For this review, take the finished solid that the model builds, in its own axes (mm). Face numbers are marked on the shaded views. A direction names the side the tool comes from. Coordinates: 2 decimals unless noted, no trailing zeros. Order: outer loops, then holes, each group sorted by start corner. A loop starts at its lowest first (then second) coordinate and runs counter-clockwise, first axis right, second up. Notation, with made-up numbers: M 37,10.5 L 59,10.5 A27 cw 59,46.5 Z; hole C 61,33 d11. An arc over 180 degrees is marked long. Use CSV: the item, a comma, the result in double quotes.
```python
from build123d import *

# Parameters (mm, degrees)
SKETCH2_R                            = 3.35
F_40_SERIES_TS40_40LM_650033_2_DEPTH = 115
M8X1_25_TAPPED_HOLE3_D               = 6.8
M8X1_25_TAPPED_HOLE3_DEPTH           = 25
M8X1_25_TAPPED_HOLE3_TIP             = 2.042926105


with BuildPart() as part:
    # Sketch2 → 40 series TS40-40LM-650033(2) (new body)
    with BuildSketch(Plane(origin=(0, 0, 0), x_dir=(-1, 0, 0), z_dir=(0, 1, 0))):
        with BuildLine():
            Line((-7.7064, 0), (-7.7064, 5.551138531))
            Line((-7.7064, 5.551138531), (-13.331261469, 11.176))
            Line((-13.331261469, 11.176), (-16.6472, 11.176))
            Line((-16.6472, 11.176), (-16.6472, 7.6835))
            Line((-16.6472, 7.6835), (-15.2502, 7.6835))
            Line((-15.2502, 7.6835), (-15.2502, 4.0005))
            Line((-15.2502, 4.0005), (-20, 4.0005))
            Line((-20, 4.0005), (-20, 16.825))
            ThreePointArc((-20, 16.825), (-19.07006403, 19.07006403), (-16.825, 20))
            Line((-16.825, 20), (-4.0005, 20))
            Line((-4.0005, 20), (-4.0005, 15.2502))
            Line((-4.0005, 15.2502), (-7.6835, 15.2502))
            Line((-7.6835, 15.2502), (-7.6835, 16.6472))
            Line((-7.6835, 16.6472), (-11.176, 16.6472))
            Line((-11.176, 16.6472), (-11.176, 13.331261469))
            Line((-11.176, 13.331261469), (-5.551138531, 7.7064))
            Line((-5.551138531, 7.7064), (0, 7.7064))
            Line((0, 7.7064), (5.551138531, 7.7064))
            Line((5.551138531, 7.7064), (11.176, 13.331261469))
            Line((11.176, 13.331261469), (11.176, 16.6472))
            Line((11.176, 16.6472), (7.6835, 16.6472))
            Line((7.6835, 16.6472), (7.6835, 15.2502))
            Line((7.6835, 15.2502), (4.0005, 15.2502))
            Line((4.0005, 15.2502), (4.0005, 20))
            Line((4.0005, 20), (16.825, 20))
            ThreePointArc((16.825, 20), (19.07006403, 19.07006403), (20, 16.825))
            Line((20, 16.825), (20, 4.0005))
            Line((20, 4.0005), (15.2502, 4.0005))
            Line((15.2502, 4.0005), (15.2502, 7.6835))
            Line((15.2502, 7.6835), (16.6472, 7.6835))
            Line((16.6472, 7.6835), (16.6472, 11.176))
            Line((16.6472, 11.176), (13.331261469, 11.176))
            Line((13.331261469, 11.176), (7.7064, 5.551138531))
            Line((7.7064, 5.551138531), (7.7064, 0))
            Line((7.7064, 0), (7.7064, -5.551138531))
            Line((7.7064, -5.551138531), (13.331261469, -11.176))
            Line((13.331261469, -11.176), (16.6472, -11.176))
            Line((16.6472, -11.176), (16.6472, -7.6835))
            Line((16.6472, -7.6835), (15.2502, -7.6835))
            Line((15.2502, -7.6835), (15.2502, -4.0005))
            Line((15.2502, -4.0005), (20, -4.0005))
            Line((20, -4.0005), (20, -16.825))
            ThreePointArc((20, -16.825), (19.07006403, -19.07006403), (16.825, -20))
            Line((16.825, -20), (4.0005, -20))
            Line((4.0005, -20), (4.0005, -15.2502))
            Line((4.0005, -15.2502), (7.6835, -15.2502))
            Line((7.6835, -15.2502), (7.6835, -16.6472))
            Line((7.6835, -16.6472), (11.176, -16.6472))
            Line((11.176, -16.6472), (11.176, -13.331261469))
            Line((11.176, -13.331261469), (5.551138531, -7.7064))
            Line((5.551138531, -7.7064), (0, -7.7064))
            Line((0, -7.7064), (-5.551138531, -7.7064))
            Line((-5.551138531, -7.7064), (-11.176, -13.331261469))
            Line((-11.176, -13.331261469), (-11.176, -16.6472))
            Line((-11.176, -16.6472), (-7.6835, -16.6472))
            Line((-7.6835, -16.6472), (-7.6835, -15.2502))
            Line((-7.6835, -15.2502), (-4.0005, -15.2502))
            Line((-4.0005, -15.2502), (-4.0005, -20))
            Line((-4.0005, -20), (-16.825, -20))
            ThreePointArc((-16.825, -20), (-19.07006403, -19.07006403), (-20, -16.825))
            Line((-20, -16.825), (-20, -4.0005))
            Line((-20, -4.0005), (-15.2502, -4.0005))
            Line((-15.2502, -4.0005), (-15.2502, -7.6835))
            Line((-15.2502, -7.6835), (-16.6472, -7.6835))
            Line((-16.6472, -7.6835), (-16.6472, -11.176))
            Line((-16.6472, -11.176), (-13.331261469, -11.176))
            Line((-13.331261469, -11.176), (-7.7064, -5.551138531))
            Line((-7.7064, -5.551138531), (-7.7064, 0))
        make_face()
        Circle(SKETCH2_R, mode=Mode.SUBTRACT)
        with BuildLine():
            Line((18.222, 12.8372), (18.222, 15.428))
            ThreePointArc((18.222, 15.428), (17.403656347, 17.403656347), (15.428, 18.222))
            Line((15.428, 18.222), (12.8372, 18.222))
            Line((12.8372, 18.222), (12.8372, 12.8372))
            Line((12.8372, 12.8372), (18.222, 12.8372))
        make_face(mode=Mode.SUBTRACT)
        with BuildLine():
            Line((12.8372, -12.8372), (18.222, -12.8372))
            Line((18.222, -12.8372), (18.222, -15.428))
            ThreePointArc((18.222, -15.428), (17.403656347, -17.403656347), (15.428, -18.222))
            Line((15.428, -18.222), (12.8372, -18.222))
            Line((12.8372, -18.222), (12.8372, -12.8372))
        make_face(mode=Mode.SUBTRACT)
        with BuildLine():
            Line((-18.222, -12.8372), (-18.222, -15.428))
            ThreePointArc((-18.222, -15.428), (-17.403656347, -17.403656347), (-15.428, -18.222))
            Line((-15.428, -18.222), (-12.8372, -18.222))
            Line((-12.8372, -18.222), (-12.8372, -12.8372))
            Line((-12.8372, -12.8372), (-18.222, -12.8372))
        make_face(mode=Mode.SUBTRACT)
        with BuildLine():
            Line((-12.8372, 12.8372), (-18.222, 12.8372))
            Line((-18.222, 12.8372), (-18.222, 15.428))
            ThreePointArc((-18.222, 15.428), (-17.403656347, 17.403656347), (-15.428, 18.222))
            Line((-15.428, 18.222), (-12.8372, 18.222))
            Line((-12.8372, 18.222), (-12.8372, 12.8372))
        make_face(mode=Mode.SUBTRACT)
    extrude(amount=F_40_SERIES_TS40_40LM_650033_2_DEPTH)

    # M8x1.25 Tapped Hole3
    with Locations(Plane(origin=(0, 0, 0), x_dir=(-1, 0, 0), z_dir=(0, -1, 0))):
        with Locations((0, 0)):
            Hole(M8X1_25_TAPPED_HOLE3_D / 2, depth=M8X1_25_TAPPED_HOLE3_DEPTH)
            with Locations((0, 0, -(M8X1_25_TAPPED_HOLE3_DEPTH + M8X1_25_TAPPED_HOLE3_TIP / 2))):  # 118° drill point
                Cone(0, M8X1_25_TAPPED_HOLE3_D / 2, M8X1_25_TAPPED_HOLE3_TIP, mode=Mode.SUBTRACT)


solid = part.part
```
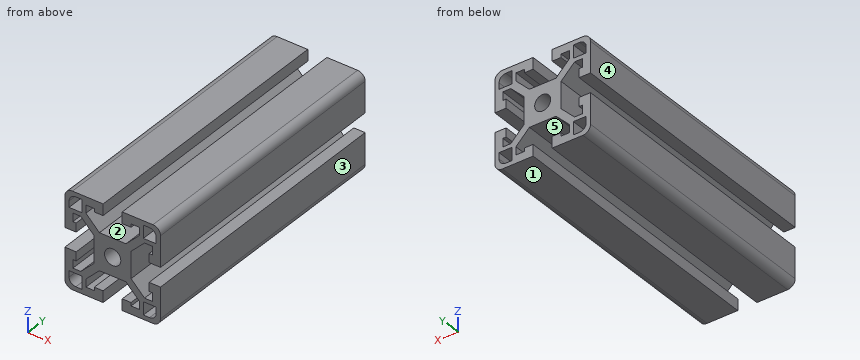
Item 1: Add section D-D on z = 10. State the section outline as (x, y) points, and give its area (3 significant figures).
Solutions:
outline,"M -20,0 L -16.65,0 L -16.65,115 L -20,115 Z; M -12.16,0 L -7.84,0 L -7.84,115 L -12.16,115 Z; M 7.84,0 L 12.16,0 L 12.16,115 L 7.84,115 Z; M 16.65,0 L 20,0 L 20,115 L 16.65,115 Z"
area,"1,760 mm^2"
Item 2: Add section A-A on z = 0. State the section outline as (x, y) points, and give its area (3 significant figures).
Solutions:
outline,"M -7.71,0 L -3.4,0 L -3.4,25 L -3.35,25.03 L -3.35,115 L -7.71,115 Z; M 3.35,25.03 L 3.4,25 L 3.4,0 L 7.71,0 L 7.71,115 L 3.35,115 Z"
area,"999 mm^2"
Item 3: For the marked faces 4 and 5, list the 3-axis set-ups (+Z, -Z, +X, -X, +Y, -Y) from which the entire face can be reached by the end or side of a thin tool; tool diameter is ignored.
Solutions:
face 4,"+Z, -Z, -X, +Y, -Y"
face 5,"+Y, -Y"
Item 4: Add section B-B on x = 0. State the section outline as (y, z) points.
Solutions:
outline,"M 0,-7.71 L 115,-7.71 L 115,-3.35 L 25.03,-3.35 L 25,-3.4 L 0,-3.4 Z; M 0,3.4 L 25,3.4 L 25.03,3.35 L 115,3.35 L 115,7.71 L 0,7.71 Z"
Item 5: Clearance check with a flat-ended pin moving along its axis: pin 1 Ø5.5 at (x, y) = (0.5, 60.5) entering from -Z. State where the tip first meets the part, or that it passes through.
Solutions:
pin 1,"z = -7.71"
Item 6: To check wall thickness, follow line 1 along X through (y, z) = (106, 15.5); line 2 along X through (y, z) = (15.5, 14.5). State the ranges of each line that lie inside material, in increasing order. Write a range as [from, to].
Solutions:
line 1,"[-20, -18.22], [-12.84, -11.18], [-7.68, -4], [4, 7.68], [11.18, 12.84], [18.22, 20]"
line 2,"[-20, -18.22], [-12.84, -11.18], [11.18, 12.84], [18.22, 20]"
Item 7: Add section C-C on y = 19. State how many separate pieces and enclosed holes the cut face has, and give its area (3 significant figures).
Solutions:
separate pieces,"1"
enclosed holes,"5"
area,"707 mm^2"
Item 8: Draft analysis for pull direction X (two halves, no side actions). For the marked faces 1, 2 and 3, state which applies: released by +X, released by -X, zero draft, split by the parting line, or undercut.
Solutions:
face 1,"zero draft"
face 2,"undercut"
face 3,"released by +X"
